```python
from build123d import *

# Parameters (mm, degrees)
CROQUIS2_R              = 1.5
SALIENTE_EXTRUIR1_DEPTH = 4
CROQUIS3_R              = 5
CORTAR_EXTRUIR1_DEPTH   = 2.5
CROQUIS6_R              = 5.5
CORTAR_EXTRUIR2_DEPTH   = 37.619666847
CHAFL_N1_SIZE           = 1
CHAFL_N2_SIZE           = 0.5


with BuildPart() as part:
    # Croquis2 → Saliente-Extruir1 (new body)
    with BuildSketch(Plane(origin=(0, 0, 0), x_dir=(1, 0, 0), z_dir=(0, 1, 0))):
        with BuildLine():
            Line((-25, 10), (25, 10))
            ThreePointArc((25, 10), (35, 0), (25, -10))
            Line((25, -10), (-25, -10))
            ThreePointArc((-25, -10), (-35, 0), (-25, 10))
        make_face()
        with Locations(Location((-25, 0, 0), (0, 0, 270))):
            Circle(CROQUIS2_R, mode=Mode.SUBTRACT)
        with Locations(Location((25, 0, 0), (0, 0, 270))):
            Circle(CROQUIS2_R, mode=Mode.SUBTRACT)
        with Locations(Location((-15, 0, 0), (0, 0, 270))):
            Circle(CROQUIS2_R, mode=Mode.SUBTRACT)
    extrude(amount=SALIENTE_EXTRUIR1_DEPTH)

    # Croquis3 → Cortar-Extruir1 (cut)
    with BuildSketch(Plane(origin=(0, 4, 0), x_dir=(1, 0, 0), z_dir=(0, 1, 0))):
        with Locations(Location((-25, 0, 0), (0, 0, 270))):
            Circle(CROQUIS3_R)
        with Locations(Location((25, 0, 0), (0, 0, 270))):
            Circle(CROQUIS3_R)
    extrude(amount=-CORTAR_EXTRUIR1_DEPTH, mode=Mode.SUBTRACT)

    # Croquis6 → Cortar-Extruir2 (cut, through all)
    with BuildSketch(Plane(origin=(0, 4, 0), x_dir=(1, 0, 0), z_dir=(0, 1, 0))):
        with Locations(Location((0, 0, 0), (0, 0, 270))):
            Circle(CROQUIS6_R)
    extrude(amount=-CORTAR_EXTRUIR2_DEPTH, mode=Mode.SUBTRACT)

    # Croquis5 → Revolución1 (revolve)
    with BuildSketch(Plane.XY, mode=Mode.PRIVATE) as revoluci_n1_sk:
        with BuildLine():
            Line((5, 4.75), (5.5, 4))
            Line((5.5, 4), (6.8125, 4))
            Line((6.8125, 4), (5, 7.75))
            Line((5, 7.75), (4, 7.75))
            ThreePointArc((4, 7.75), (4.74341649, 6.33113883), (5, 4.75))
        make_face()
    revolve(revoluci_n1_sk.sketch.rotate(Axis((0, -0.25, 0), (0, 1, 0)), 90), axis=Axis((0, -0.25, 0), (0, 1, 0)))

    # Chaflán1
    chafl_n1_edges = [part.edges().sort_by_distance(p)[0] for p in [
        (-15, 0, -1.5),
        (-15, 4, -1.5),
    ]]
    chamfer(chafl_n1_edges, length=CHAFL_N1_SIZE)

    # Chaflán2
    chafl_n2_edges = [part.edges().sort_by_distance(p)[0] for p in [
        (35, 4, 0),
        (0, 4, -10),
        (-25, 4, -5),
        (25, 4, -5),
        (-35, 4, 0),
        (0, 0, -10),
        (35, 0, 0),
        (0, 0, 10),
        (-35, 0, 0),
        (0, 4, 10),
    ]]
    chamfer(chafl_n2_edges, length=CHAFL_N2_SIZE)


solid = part.part
```
Read the model definition and answer for the solid it produces. Units are mm, in the model's axes. A direction names the side the tool comes from. Give positions to 0.01 mm unless a question says otherwise; leave off trailing zeros. Write each loop counter-clockwise with the first axis right and the second up, starting at its lowest first coordinate (ties: lowest second). Pieces come first, ordered by that corner, then holes. Notation, with made-up numbers: (10.25, 63) -> (23.25, 63) arc R5 ccw to (23.25, 71) -> close; hole circle Ø2 at (50.25, -11). An arc over 180 degrees is marked (long way). Answer as a JSON object with one key per item and string values.
1) For a pull along X with two mould halves and no side action, classify faces 4 (the cylindrical face through (-14.55, 1.99, 1.43)), 5 (the flat face through (0, 2, -10)), 6 (the cylindrical face through (-29.88, 2.51, -1.08)), 7 (the cylindrical face through (35, 2, 0)) as pulls with the +X half, pulls with the -X half, needs draft (parallel to the pull), parting line crosses it, or undercut.
Findings below:
{"face 4": "undercut", "face 5": "needs draft", "face 6": "undercut", "face 7": "pulls with the +X half"}
2) Straight lines are drawn through the part: probe 1 along X at (y, z) = (2, 0); probe 2 along X at (y, z) = (1.05, 0); probe 3 along Y at (x, z) = (12.5, 1.25). For each, find the intervals that lie inside material, in ascending order. Write a range as from..to.
Findings below:
{"probe 1": "x = -35..-30, -20..-16.5, -13.5..-5.5, 5.5..20, 30..35", "probe 2": "x = -35..-26.5, -23.5..-16.5, -13.5..-5.5, 5.5..23.5, 26.5..35", "probe 3": "y = 0..4"}
3) Section C-C on z = 0 is taken. Count the separate pieces of the cut face and the enclosed holes in it, then the cut area to 3 significant figures.
Findings below:
{"separate pieces": "5", "enclosed holes": "0", "area": "170 mm^2"}
4) Flat-ended cylindrical pins translate along their axes: pin 1 Ø11 at (x, z) = (-26.5, -2) entering from +Y; pin 2 Ø9 at (x, z) = (0, 0) entering from -Y. Find the tip coordinate at first contact, or state that the pin passes through.
Findings below:
{"pin 1": "stops at y = 4", "pin 2": "stops at y = 6.93"}
5) Section B-B on x = -15 is taken. Write down the section's boundary in (y, z), then the cut area to 3 significant figures.
Findings below:
{"outline": "(0, -9.5) -> (0.5, -10) -> (3.5, -10) -> (4, -9.5) -> (4, -2.5) -> (3, -1.5) -> (1, -1.5) -> (0, -2.5) -> close; (0, 2.5) -> (1, 1.5) -> (3, 1.5) -> (4, 2.5) -> (4, 9.5) -> (3.5, 10) -> (0.5, 10) -> (0, 9.5) -> close", "area": "65.5 mm^2"}
6) A tool of negligible diameter and unlimited length cuts with its end or side. For faces 1 (the cylindrical face through (20.12, 2.51, -1.08)), 2 (the cylindrical face through (-5.37, 2.03, -1.19)), 3 (the conical face through (-34.633, 3.865, 0.212)), from which of +Z, -Z, +X, -X, +Y, -Y can it reach the whole face along a straight path? Write none if from no direction.
Findings below:
{"face 1": "+Y", "face 2": "-Y", "face 3": "-X, +Y"}
7) Section D-D on y = 6 is taken. Write down the section's boundary in (x, z), then the cut area to 3 significant figures.
Findings below:
{"outline": "circle Ø11.69 at (0, 0); hole circle Ø9.68 at (0, 0)", "area": "33.7 mm^2"}
8) Section A-A on x = 0 is taken. Write down the section's boundary in (y, z).
Findings below:
{"outline": "(0, -9.5) -> (0.5, -10) -> (3.5, -10) -> (4, -9.5) -> (4, -6.81) -> (7.75, -5) -> (7.75, -4) arc R5 cw to (4.75, -5) -> (4, -5.5) -> (0, -5.5) -> close; (0, 5.5) -> (4, 5.5) -> (4.75, 5) arc R5 cw to (7.75, 4) -> (7.75, 5) -> (4, 6.81) -> (4, 9.5) -> (3.5, 10) -> (0.5, 10) -> (0, 9.5) -> close"}
